from build123d import *

# Parameters (mm, degrees)
SKETCH1_W           = 126.5
SKETCH1_H           = 100
SKETCH1_H_2         = 5
BOSS_EXTRUDE1_DEPTH = 5
BOSS_EXTRUDE2_DEPTH = 4
BOSS_EXTRUDE3_DEPTH = 2
SKETCH3_R           = 3.5
SKETCH3_R_2         = 1.475
BOSS_EXTRUDE4_DEPTH = 2.5
CUT_EXTRUDE1_START  = -2.5
SKETCH3_6_R         = 1.25
SKETCH3_6_R_2       = 1.475
CUT_EXTRUDE1_DEPTH  = 2.5


with BuildPart() as part:
    # Sketch1 → Boss-Extrude1 (new body)
    with BuildSketch(Plane(origin=(0, 0, 0), x_dir=(1, 0, 0), z_dir=(0, 1, 0))):
        Rectangle(SKETCH1_W, SKETCH1_H)
        Polygon((63.25, 50), (63.25, -50), (63.25, -55), (68.25, -55), (68.25, 55), (-68.25, 55), (-68.25, -55), (-63.25, -55), (-63.25, -50), (-63.25, 50), align=None)
        with Locations((0, -52.5)):
            Rectangle(SKETCH1_W, SKETCH1_H_2)
    extrude(amount=BOSS_EXTRUDE1_DEPTH)

    # Sketch1_4 → Boss-Extrude2 (add)
    with BuildSketch(Plane(origin=(0, 0, 0), x_dir=(1, 0, 0), z_dir=(0, 1, 0))):
        Polygon((63.25, 50), (63.25, -50), (63.25, -55), (68.25, -55), (68.25, 55), (-68.25, 55), (-68.25, -55), (-63.25, -55), (-63.25, -50), (-63.25, 50), align=None)
    extrude(amount=-BOSS_EXTRUDE2_DEPTH)

    # Sketch2 → Boss-Extrude3 (add)
    with BuildSketch(Plane.XZ.offset(4)):
        Polygon((-60.25, 55), (-60.25, -47), (60.25, -47), (60.25, 55), (63.25, 55), (63.25, -50), (-63.25, -50), (-63.25, 55), align=None)
    extrude(amount=-BOSS_EXTRUDE3_DEPTH)

    # Sketch3 → Boss-Extrude4 (add)
    # profile 1 of 8: a face of its own
    with BuildSketch(Plane(origin=(0, 5, 0), x_dir=(1, 0, 0), z_dir=(0, 1, 0))):
        with Locations(Location((29, -51.5, 0), (0, 0, 270))):
            Circle(SKETCH3_R)
        with Locations(Location((29, -51.5, 0), (0, 0, 270))):
            Circle(SKETCH3_R_2, mode=Mode.SUBTRACT)
    # profile 2 of 8: a face of its own
    with BuildSketch(Plane(origin=(0, 5, 0), x_dir=(1, 0, 0), z_dir=(0, 1, 0))):
        with Locations(Location((29, -28.5, 0), (0, 0, 270))):
            Circle(SKETCH3_R)
        with Locations(Location((29, -28.5, 0), (0, 0, 270))):
            Circle(SKETCH3_R_2, mode=Mode.SUBTRACT)
    # profile 3 of 8: a face of its own
    with BuildSketch(Plane(origin=(0, 5, 0), x_dir=(1, 0, 0), z_dir=(0, 1, 0))):
        with Locations(Location((-29, -51.5, 0), (0, 0, 270))):
            Circle(SKETCH3_R)
        with Locations(Location((-29, -51.5, 0), (0, 0, 270))):
            Circle(SKETCH3_R_2, mode=Mode.SUBTRACT)
    # profile 4 of 8: a face of its own
    with BuildSketch(Plane(origin=(0, 5, 0), x_dir=(1, 0, 0), z_dir=(0, 1, 0))):
        with Locations(Location((-29, -28.5, 0), (0, 0, 270))):
            Circle(SKETCH3_R)
        with Locations(Location((-29, -28.5, 0), (0, 0, 270))):
            Circle(SKETCH3_R_2, mode=Mode.SUBTRACT)
    # profile 5 of 8: a face of its own
    with BuildSketch(Plane(origin=(0, 5, 0), x_dir=(1, 0, 0), z_dir=(0, 1, 0))):
        with Locations(Location((64.421406537, 51.425448186, 0), (0, 0, 270))):
            Circle(SKETCH3_R)
        with Locations(Location((64.421406537, 51.425448186, 0), (0, 0, 270))):
            Circle(SKETCH3_R_2, mode=Mode.SUBTRACT)
    # profile 6 of 8: a face of its own
    with BuildSketch(Plane(origin=(0, 5, 0), x_dir=(1, 0, 0), z_dir=(0, 1, 0))):
        with Locations(Location((41.421406537, 51.425448186, 0), (0, 0, 270))):
            Circle(SKETCH3_R)
        with Locations(Location((41.421406537, 51.425448186, 0), (0, 0, 270))):
            Circle(SKETCH3_R_2, mode=Mode.SUBTRACT)
    # profile 7 of 8: a face of its own
    with BuildSketch(Plane(origin=(0, 5, 0), x_dir=(1, 0, 0), z_dir=(0, 1, 0))):
        with Locations(Location((64.421406537, -6.574551814, 0), (0, 0, 270))):
            Circle(SKETCH3_R)
        with Locations(Location((64.421406537, -6.574551814, 0), (0, 0, 270))):
            Circle(SKETCH3_R_2, mode=Mode.SUBTRACT)
    # profile 8 of 8: a face of its own
    with BuildSketch(Plane(origin=(0, 5, 0), x_dir=(1, 0, 0), z_dir=(0, 1, 0))):
        with Locations(Location((41.421406537, -6.574551814, 0), (0, 0, 270))):
            Circle(SKETCH3_R)
        with Locations(Location((41.421406537, -6.574551814, 0), (0, 0, 270))):
            Circle(SKETCH3_R_2, mode=Mode.SUBTRACT)
    extrude(amount=BOSS_EXTRUDE4_DEPTH)

    # Sketch3_6 → Cut-Extrude1 (cut)
    # profile 1 of 5: a face of its own
    with BuildSketch(Plane(origin=(0, 5, 0), x_dir=(1, 0, 0), z_dir=(0, 1, 0)).offset(CUT_EXTRUDE1_START)):
        with Locations(Location((-29, -51.5, 0), (0, 0, 270))):
            Circle(SKETCH3_6_R)
    # profile 2 of 5: a face of its own
    with BuildSketch(Plane(origin=(0, 5, 0), x_dir=(1, 0, 0), z_dir=(0, 1, 0)).offset(CUT_EXTRUDE1_START)):
        with Locations(Location((-29, -28.5, 0), (0, 0, 270))):
            Circle(SKETCH3_6_R)
    # profile 3 of 5: a face of its own
    with BuildSketch(Plane(origin=(0, 5, 0), x_dir=(1, 0, 0), z_dir=(0, 1, 0)).offset(CUT_EXTRUDE1_START)):
        with Locations(Location((29, -28.5, 0), (0, 0, 270))):
            Circle(SKETCH3_6_R)
    # profile 4 of 5: a face of its own
    with BuildSketch(Plane(origin=(0, 5, 0), x_dir=(1, 0, 0), z_dir=(0, 1, 0)).offset(CUT_EXTRUDE1_START)):
        with Locations(Location((29, -51.5, 0), (0, 0, 270))):
            Circle(SKETCH3_6_R)
    # profile 5 of 5: a face of its own
    with BuildSketch(Plane(origin=(0, 5, 0), x_dir=(1, 0, 0), z_dir=(0, 1, 0)).offset(CUT_EXTRUDE1_START)):
        with Locations(Location((64.421406537, 51.425448186, 0), (0, 0, 270))):
            Circle(SKETCH3_6_R_2)
        with Locations(Location((64.421406537, 51.425448186, 0), (0, 0, 270))):
            Circle(SKETCH3_6_R, mode=Mode.SUBTRACT)
    extrude(amount=CUT_EXTRUDE1_DEPTH, mode=Mode.SUBTRACT)


solid = part.part
Part model, mm, in its own coordinate system. A direction names the side the tool comes from. Give positions to 0.01 mm unless a question says otherwise; leave off trailing zeros. Write each loop counter-clockwise with the first axis right and the second up, starting at its lowest first coordinate (ties: lowest second). Pieces come first, ordered by that corner, then holes.
1) Cut at B-B on x = -19. Write the cut outline in (y, z), then the cut area to 3 significant figures.
Resolved:
outline: (-4, -55) - (5, -55) - (5, 55) - (0, 55) - (0, -50) - (-2, -50) - (-2, -47) - (-4, -47) - close
area: 576 mm2
2) Probe L1, parallel to X at y = 6.7, z = 51.5 (3 decimals); L2, parallel to X at y = 4.35, z = 51.5; L3, parallel to X at y = -1, z = -9.5. List the from-to ranges inside material, lowest first.
Resolved:
L1: x = -32.5 to -30.475, -27.525 to -25.5, 25.5 to 27.525, 30.475 to 32.5
L2: x = -68.25 to -30.25, -27.75 to 27.75, 30.25 to 68.25
L3: x = -68.25 to -63.25, 63.25 to 68.25
3) Which spindle directions (+Z, -Z, +X, -X, +Y, -Y) get a long thin tool onto all of the face, cutting with end or side? Do faces 1 (the face through (-31, 7.5, 51)), 2 (the face through (31.365, 6.232, 48.92)). Say none if no direction does.
Resolved:
face 1: +Z, -Z, +X, -X, +Y
face 2: +Y
4) Two-plate mould, pull along Z, no slides. Class faces 3 (the face through (62.9, 7.5, -50.7)), 4 (the face through (63.86, 4.96, -50.06)): released by +Z, released by -Z, zero draft, split by the parting line, or undercut.
Resolved:
face 3: zero draft
face 4: undercut
5) Pin check, flat tips, straight feed: pin 1 (2 mm diameter, centred on x = -14.5, z = 39.5, fed in from -Y); pin 2 (0.9 mm diameter, centred on x = -29, z = 28, fed in from +Y); pin 3 (8 mm diameter, centred on x = 15, z = -11.5, fed in from +Y). Stop position of each tip, or through.
Resolved:
pin 1: stops at y = 0
pin 2: stops at y = 2.5
pin 3: stops at y = 5
6) Cut at A-A on z = 1. Write the cut outline in (x, y).
Resolved:
outline: (-68.25, -4) - (-60.25, -4) - (-60.25, -2) - (-63.25, -2) - (-63.25, 0) - (63.25, 0) - (63.25, -2) - (60.25, -2) - (60.25, -4) - (68.25, -4) - (68.25, 5) - (-68.25, 5) - close
